```python
from build123d import *
from build123d.topology import SkipClean

# Parameters (mm, degrees)
SKETCH1_R                       = 2.5
BOSS_EXTRUDE1_DEPTH             = 8
SKETCH2_R                       = 0.8
SCREW_HOLES_DEPTH               = 52.103203384
SKETCH10_R                      = 1.25
SCREW_HEADS_DEPTH               = 2
DISTAL_MIDDLE_START             = 3
DISTAL_MIDDLE_CABLE_CANAL_DEPTH = 5
POT_START                       = 8
POT_INSERT_DEPTH                = 2.5
CUT_EXTRUDE1_START              = 3
CUT_EXTRUDE1_OUTLINE_R          = 0.8
CUT_EXTRUDE1_DEPTH              = 5
SKETCH7_R                       = 7.5
CUT_EXTRUDE2_DEPTH              = 4


# Read off the part's stored shape, not the designer's step: Cut-Extrude1
with BuildPart() as part:
    # Sketch1 → Boss-Extrude1 (new body)
    with BuildSketch(Plane(origin=(0, 0, 0), x_dir=(1, 0, 0), z_dir=(0, 1, 0))):
        with BuildLine():
            Line((13, 10), (13, -10))
            Line((13, -10), (17, -10))
            Line((17, -10), (17, -12.105263158))
            Line((17, -12.105263158), (38, -11))
            ThreePointArc((38, -11), (49, 0), (38, 11))
            Line((38, 11), (17, 12.105263158))
            Line((17, 12.105263158), (17, 10))
            Line((17, 10), (13, 10))
        make_face()
        with Locations(Location((38, 0, 0), (0, 0, 270))):
            Circle(SKETCH1_R, mode=Mode.SUBTRACT)
    extrude(amount=BOSS_EXTRUDE1_DEPTH)

    # Sketch2 → Screw Holes (cut, through all)
    with BuildSketch(Plane(origin=(0, 0, 0), x_dir=(1, 0, 0), z_dir=(0, 1, 0))):
        with Locations(Location((24, 8.5, 0), (0, 0, 270))):
            Circle(SKETCH2_R)
        with Locations(Location((24, 0, 0), (0, 0, 270))):
            Circle(SKETCH2_R)
        with Locations(Location((24, -8.5, 0), (0, 0, 270))):
            Circle(SKETCH2_R)
    extrude(amount=SCREW_HOLES_DEPTH, mode=Mode.SUBTRACT)

    # Sketch10 → Screw Heads (cut)
    with BuildSketch(Plane(origin=(0, 0, 0), x_dir=(1, 0, 0), z_dir=(0, 1, 0))):
        with Locations(Location((24, 0, 0), (0, 0, 270))):
            Circle(SKETCH10_R)
    extrude(amount=SCREW_HEADS_DEPTH, mode=Mode.SUBTRACT)

    # Sketch 3 → Distal_Middle Cable Canal (cut)
    with SkipClean():  # the faces are left unmerged after this step: merging them gives an invalid solid
        with BuildSketch(Plane(origin=(0, 0, 0), x_dir=(1, 0, 0), z_dir=(0, 1, 0)).offset(DISTAL_MIDDLE_START)):
            with BuildLine():
                Line((19, 5), (13, 5))
                Line((13, 5), (13, 3))
                Line((13, 3), (19, 3))
                Line((19, 3), (20.058874503, 3))
                ThreePointArc((20.058874503, 3), (25.033759124, 3.989566077), (29.251262658, 6.807611845))
                Line((29.251262658, 6.807611845), (30.221825407, 7.778174593))
                ThreePointArc((30.221825407, 7.778174593), (33.790482244, 10.162674858), (38, 11))
                Line((38, 11), (31.634673214, 11.335017199))
                ThreePointArc((31.634673214, 11.335017199), (30.147717634, 10.360582109), (28.807611845, 9.192388155))
                Line((28.807611845, 9.192388155), (28.422835534, 8.807611845))
                ThreePointArc((28.422835534, 8.807611845), (24.205331999, 5.989566077), (19.230447378, 5))
                Line((19.230447378, 5), (19, 5))
            make_face()
            with BuildLine():
                Line((19, -5), (13, -5))
                Line((13, -5), (13, -3))
                Line((13, -3), (19, -3))
                Line((19, -3), (20.058874503, -3))
                ThreePointArc((20.058874503, -3), (25.033759124, -3.989566077), (29.251262658, -6.807611845))
                Line((29.251262658, -6.807611845), (30.221825407, -7.778174593))
                ThreePointArc((30.221825407, -7.778174593), (33.790482244, -10.162674858), (38, -11))
                Line((38, -11), (31.634673214, -11.335017199))
                ThreePointArc((31.634673214, -11.335017199), (30.147717634, -10.360582109), (28.807611845, -9.192388155))
                Line((28.807611845, -9.192388155), (28.422835534, -8.807611845))
                ThreePointArc((28.422835534, -8.807611845), (24.205331999, -5.989566077), (19.230447378, -5))
                Line((19.230447378, -5), (19, -5))
            make_face()
        extrude(amount=DISTAL_MIDDLE_CABLE_CANAL_DEPTH, mode=Mode.SUBTRACT)

    # Sketch3 → Pot Insert (cut)
    with SkipClean():  # the faces are left unmerged after this step: merging them gives an invalid solid
        with BuildSketch(Plane(origin=(28.28760271, 0, 0), x_dir=(1, 0, 0), z_dir=(0, 1, 0)).offset(POT_START)):
            Polygon((16.71239729, 0), (16.71239729, 1.5), (15.21239729, 1.5), (13.71239729, 4.5), (13.71239729, 5.5), (9.71239729, 5.5), (5.46239729, 5.5), (5.46239729, 4.5), (0.21239729, 4.5), (0.21239729, 0), (0.21239729, -4.5), (5.46239729, -4.5), (5.46239729, -5.5), (9.71239729, -5.5), (13.71239729, -5.5), (13.71239729, -4.5), (15.21239729, -1.5), (16.71239729, -1.5), align=None)
        extrude(amount=-POT_INSERT_DEPTH, mode=Mode.SUBTRACT)

    # Cut-Extrude1 outline → Cut-Extrude1 (cut)
    with SkipClean():  # the faces are left unmerged after this step: merging them gives an invalid solid
        with BuildSketch(Plane(origin=(0, 0, 0), x_dir=(1, 0, 0), z_dir=(0, 1, 0)).offset(CUT_EXTRUDE1_START)):
            with BuildLine():
                Line((13, -1), (21.267949192, -1))
                ThreePointArc((21.267949192, -1), (22, -1.732050808), (23, -2))
                Line((23, -2), (24, -2))
                ThreePointArc((24, -2), (26, 0), (24, 2))
                Line((24, 2), (23, 2))
                ThreePointArc((23, 2), (22, 1.732050808), (21.267949192, 1))
                Line((21.267949192, 1), (13, 1))
                Line((13, 1), (13, -1))
            make_face()
            with Locations((24, 0)):
                Circle(CUT_EXTRUDE1_OUTLINE_R, mode=Mode.SUBTRACT)
        extrude(amount=CUT_EXTRUDE1_DEPTH, mode=Mode.SUBTRACT)

    # Sketch7 → Cut-Extrude2 (cut)
    with SkipClean():  # the faces are left unmerged after this step: merging them gives an invalid solid
        with BuildSketch(Plane(origin=(0, 0, 0), x_dir=(1, 0, 0), z_dir=(0, 1, 0))):
            with Locations(Location((38, 0, 0), (0, 0, 270))):
                Circle(SKETCH7_R)
        extrude(amount=CUT_EXTRUDE2_DEPTH, mode=Mode.SUBTRACT)


solid = part.part
```
Design review of the part built by this model. Coordinates are the model's own, in mm. A direction names the side the tool comes from. Round coordinates to 2 decimals unless told otherwise and drop trailing zeros. Write each loop counter-clockwise with the first axis right and the second up, starting at its lowest first coordinate (ties: lowest second). Pieces come first, ordered by that corner, then holes. Notation, with made-up numbers: (-8, 72.5) -> (16, 72.5) arc R18 ccw to (16, 107.5) -> close; hole circle Ø5 at (-39.5, 84.25). An arc over 180 degrees is marked (long way). Write item = value, one per line. Start each with the question number.
1) Wall thickness on probe 1 along X at (y, z) = (0.75, 0); probe 2 along X at (y, z) = (0.75, 1); probe 3 along Z at (x, y) = (38, 4.65): over which ranges is each line inside the solid? List them lowest first. Write a range as from..to.
2) Take a section at C-C, the plane z = -10.5. State the section outline as (x, y) points, plus the area to 3 significant figures.
3) Take a section at B-B, the plane x = 40. State the section outline as (y, z) points.
4) Take a section at A-A, the plane y = 6. Count the separate pieces of the cut face and the enclosed holes in it, plus the area to 3 significant figures.
5) Clearance check with flat-ended pins moving along their axes: pin 1 (3 mm diameter, centred on x = 29.5, y = 1.5, fed in from +Z); pin 2 (4 mm diameter, centred on x = 16.5, y = 5.5, fed in from -Z); pin 3 (2.5 mm diameter, centred on x = 15.5, y = 6.5, fed in from +Z); pin 4 (1.5 mm diameter, centred on x = 35, y = 5, fed in from -Z). State where each tip first meets the part, or that it passes through.
6) Take a section at D-D, the plane x = 18. State the section outline as (y, z) points.
7) Mouldability with a two-part tool opening along X and no side actions: class faces 4 (the face through (17, 4, 11)), 5 (the face through (22.01, 5.46, -1.74)), 6 (the face through (17, 5, -1)), 7 (the face through (24, 3.9, -9.3)) as +X half, -X half, draft (parallel to the pull), parting line (faces both ways), or undercut.
8) Tool access review of faces 1 (the face through (35.56, 4.74, -0.54)), 2 (the face through (24.271, 5.465, -6.017)), 3 (the face through (17, 5, 1)): name each direction out of +Z, -Z, +X, -X, +Y, -Y from which nothing blocks a thin tool from reaching the whole face with its end or side.
Results list:
q1.probe_1 = 13..22.75, 25.25..30.5, 45.5..49
q1.probe_2 = 13..23.25, 24.75..30.57, 45.43..48.95
q1.probe_3 = -11..-2.5, 2.5..11
q2.outline = (17, 0) -> (41.28, 0) -> (41.28, 8) -> (34.72, 8) -> (34.72, 3) -> (30.34, 3) -> (30.34, 8) -> (17, 8) -> close
q2.area = 172 mm²
q3.outline = (0, -10.82) -> (8, -10.82) -> (8, -5.5) -> (5.5, -5.5) -> (5.5, -1.5) -> (4, -1.5) -> (4, -7.23) -> (0, -7.23) -> close; (0, 7.23) -> (4, 7.23) -> (4, 1.5) -> (5.5, 1.5) -> (5.5, 5.5) -> (8, 5.5) -> (8, 10.82) -> (0, 10.82) -> close
q4.separate_pieces = 3
q4.enclosed_holes = 3
q4.area = 472 mm²
q5.pin_1 = 11.53
q5.pin_2 = -12.11
q5.pin_3 = 10
q5.pin_4 = -10.77
q6.outline = (0, -12.05) -> (8, -12.05) -> (8, -5) -> (3, -5) -> (3, -3) -> (8, -3) -> (8, -1) -> (3, -1) -> (3, 1) -> (8, 1) -> (8, 3) -> (3, 3) -> (3, 5) -> (8, 5) -> (8, 12.05) -> (0, 12.05) -> close
q7.face_4 = -X half
q7.face_5 = undercut
q7.face_6 = draft
q7.face_7 = undercut
q8.face_1 = +Y, -Y
q8.face_2 = +Y
q8.face_3 = -X, +Y
